Verification items for the finished model (mm, model axes). A direction names the side the tool comes from. Coordinates: 2 decimals unless noted, no trailing zeros. Loops run counter-clockwise (first coordinate to the right, second up) from the corner with the lowest first, then second, coordinate; pieces in that order, holes last. Notation, with made-up numbers: (49.5, 13) -> (105.5, 13) arc R25 ccw to (105.5, 46) -> close; hole circle Ø4 at (6.25, 38.5). An arc over 180 degrees is marked (long way). Answer as a JSON object with one key per item and string values. Group by question number.
Q1. Cross-section at D-D on z = -0.5. Record the boundary of the cut face in (x, y).
Q2. Scan lines: L1, parallel to Z at x = 2.5, y = 5; L2, parallel to Z at x = 5.75, y = -4; L3, parallel to X at y = 1, z = -28.5. Record each from-to range of solid material in increasing order.
Q3. Release check for a two-part mould opening along Z. For faces 6 (the flat face through (-5, 3, 0)), 7 (the flat face through (-3, -3, -37.6)), 8 (the cylindrical face through (3.434, 1.081, -16.772)), 9 (the cylindrical face through (-5.203, -1.155, -0.493)) record: released by +Z, released by -Z, zero draft, split by the parting line, or undercut.
Q4. Set-up check for faces 1 (the cylindrical face through (1.9, 6.04, -15.8)), 2 (the conical face through (-3.822, -4.985, -36.42)), 3 (the flat face through (-3, 3, 3.48)), 4 (the cylindrical face through (-7.81, -1.73, -32.79)), 5 (the flat face through (-5, -3, -1)): record each of +Z, -Z, +X, -X, +Y, -Y from which the full face is reachable in a straight line by a thin tool's end or side.
Q5. Cross-section at A-A on y = 0. Record the boundary of the cut face in (x, z).
Q6. Gauge pin test, flat ends, axial feed: pin 1 Ø1.5 at (y, z) = (-5.5, -1.5) entering from +X; pin 2 Ø3 at (x, z) = (-6, -31) entering from +Y; pin 3 Ø8 at (y, z) = (1.5, -9.5) entering from -X; pin 4 Ø5 at (x, y) = (1.5, 2.5) entering from -Z. Record the tip position at first contact, or that the pin passes through.
Q7. Cross-section at C-C on z = -29. Record the boundary of the cut face in (x, y).
```python
from build123d import *

# Parameters (mm, degrees)
F2_R     = 3.6
F3_DEPTH = 41.081


with BuildPart() as f1:
    # F0 (on Right) → F1 (revolve)
    with BuildSketch(Plane.YZ):
        Polygon((6.33, 3.48), (0, 3.48), (0, -37.6), (6.25, -37.6), (6.33, -34.62), (8, -34.62), (8, -31.02), (6.33, -31.02), (6.33, -1), (5.33, -1), (5.33, 0), (6.33, 0), align=None)
    revolve(axis=Axis((0, 0, -17.06), (0, 0, -1)))

    # F2 (on face) → F3 (cut, through all)
    with BuildSketch(Plane.XY.offset(3.48)):
        Circle(F2_R)
    extrude(amount=-F3_DEPTH, mode=Mode.SUBTRACT)


solid = f1.part
```
Computed values:
{
 "1": {"outline": "circle Ø10.66 at (0, 0); hole circle Ø7.2 at (0, 0)"},
 "2": {"L1": "z = -37.6 to -1, 0 to 3.48", "L2": "z = -34.62 to -31.02", "L3": "x = -6.25 to -3.46, 3.46 to 6.25"},
 "3": {"face 6": "undercut", "face 7": "released by -Z", "face 8": "zero draft", "face 9": "undercut"},
 "4": {"face 1": "+Z", "face 2": "-Z", "face 3": "+Z, +X, -X, +Y, -Y", "face 4": "+Z, -Z", "face 5": "none"},
 "5": {"outline": "(-8, -34.62) -> (-6.33, -34.62) -> (-6.25, -37.6) -> (-3.6, -37.6) -> (-3.6, 3.48) -> (-6.33, 3.48) -> (-6.33, 0) -> (-5.33, 0) -> (-5.33, -1) -> (-6.33, -1) -> (-6.33, -31.02) -> (-8, -31.02) -> close; (3.6, -37.6) -> (6.25, -37.6) -> (6.33, -34.62) -> (8, -34.62) -> (8, -31.02) -> (6.33, -31.02) -> (6.33, -1) -> (5.33, -1) -> (5.33, 0) -> (6.33, 0) -> (6.33, 3.48) -> (3.6, 3.48) -> close"},
 "6": {"pin 1": "stops at x = 4.18", "pin 2": "stops at y = 6.61", "pin 3": "stops at x = -6.33", "pin 4": "stops at z = -37.6"},
 "7": {"outline": "circle Ø12.66 at (0, 0); hole circle Ø7.2 at (0, 0)"}
}
